Build history of the part. All positions in model axes, mm. A direction names the side the tool comes from. Round coordinates to 2 decimals unless told otherwise and drop trailing zeros. Loops run counter-clockwise (first coordinate to the right, second up) from the corner with the lowest first, then second, coordinate; pieces in that order, holes last. Notation, with made-up numbers: (20, 69.25) - (37, 69.25) arc R26 cw to (37, 107.25) - close; hole circle Ø7 at (83.5, 10). An arc over 180 degrees is marked (long way). Put each result on its own line as item: value. Start each with the question number.
from build123d import *

# Parameters (mm, degrees)
F0_R     = 5
F1_DEPTH = 100
F2_R     = 7.5
F2_R_2   = 5
F3_DEPTH = 20
F4_R     = 7.5
F4_R_2   = 5
F5_DEPTH = 25


with BuildPart() as f1:
    # F0 (on Front) → F1 (new body)
    with BuildSketch(Plane.XZ):
        Circle(F0_R)
    extrude(amount=F1_DEPTH)

    # F2 (on face) → F3 (join)
    with BuildSketch(Plane.XZ.offset(100)):
        Circle(F2_R)
        Circle(F2_R_2, mode=Mode.SUBTRACT)
        Circle(F2_R_2)
    extrude(amount=F3_DEPTH)

    # F4 (on face) → F5 (join)
    with BuildSketch(Plane(origin=(0, 0, 0), x_dir=(-1, 0, 0), z_dir=(0, 1, 0))):
        Circle(F4_R)
        Circle(F4_R_2, mode=Mode.SUBTRACT)
        Circle(F4_R_2)
    extrude(amount=F5_DEPTH)


solid = f1.part
1) Pull direction Y, two halves, no side cores. Call faces 3 (the face through (-7.493, -109.86, 0.33)), 4 (the face through (-1.08, -49.3, -4.88)), 5 (the face through (0, 25, 0)): pulls with the +Y half, pulls with the -Y half, needs draft (parallel to the pull), parting line crosses it, or undercut.
2) Slice it at B-B, the plane z = 0. Write the cut outline in (x, y).
3) Drill centre lines: line 1 (Y direction, x = 5, z = 4); line 2 (Z direction, x = 0.5, y = -31). Where is each one in solid material? Low to high. Write a range as [from, to].
4) Drop flat-ended pins along their axis: pin 1 Ø2 at (y, z) = (3, 5) entering from -X; pin 2 Ø1.5 at (x, y) = (-4, 7) entering from -Z; pin 3 Ø5 at (x, y) = (0, -64) entering from -Z. Give the stop position or say it passes through.
5) Which spindle directions (+Z, -Z, +X, -X, +Y, -Y) get a long thin tool onto all of the face, cutting with end or side? Do faces 1 (the face through (0, -120, 0)), 2 (the face through (2, -100, -5)). Say none if no direction does.
6) Slice it at D-D, the plane y = -104. Write the cut outline in (x, z), and give its area (3 significant figures).
7) Slice it at C-C, the plane y = -48.5. Write the cut outline in (x, z).
8) Slice it at A-A, the plane x = 0. Write the cut outline in (y, z), and give its area (4 significant figures).
Taken from the geometry:
1. face 3: needs draft
1. face 4: undercut
1. face 5: pulls with the +Y half
2. outline: (-7.5, -120) - (7.5, -120) - (7.5, -100) - (5, -100) - (5, 0) - (7.5, 0) - (7.5, 25) - (-7.5, 25) - (-7.5, 0) - (-5, 0) - (-5, -100) - (-7.5, -100) - close
3. line 1: y = [-120, -100], [0, 25]
3. line 2: z = [-4.97, 4.97]
4. pin 1: stops at x = -6.34
4. pin 2: stops at z = -6.76
4. pin 3: stops at z = -5
5. face 1: +Z, -Z, +X, -X, -Y
5. face 2: none
6. outline: circle Ø15 at (0, 0)
6. area: 177 mm2
7. outline: circle Ø10 at (0, 0)
8. outline: (-120, -7.5) - (-100, -7.5) - (-100, -5) - (0, -5) - (0, -7.5) - (25, -7.5) - (25, 7.5) - (0, 7.5) - (0, 5) - (-100, 5) - (-100, 7.5) - (-120, 7.5) - close
8. area: 1,675 mm2
